Can you work these out from the model? Positions are in its coordinate system, mm. A direction names the side the tool comes from. Give positions to 0.01 mm unless a question says otherwise; leave off trailing zeros. Write each loop counter-clockwise with the first axis right and the second up, starting at its lowest first coordinate (ties: lowest second). Pieces come first, ordered by that corner, then holes. Notation, with made-up numbers: (26, 10) -> (73, 10) arc R10 ccw to (73, 28) -> close; hole circle Ø6 at (-7.5, 48). An arc over 180 degrees is marked (long way). Answer as CSV lines item,"result". Start each with the question number.
1. I need wall thicknesses on line 1 (X direction, y = -6.5, z = 0.5); line 2 (X direction, y = -3.25, z = 101.5); line 3 (Z direction, x = -153, y = -7.5). Which ranges of each line are inside material? Lowest first, please. Write a range as [from, to].
2. If we mould it in two halves opening along Z, with no side actions, what happens to faces 5 (the face through (-297, -6, 162)), 6 (the face through (-451.677, -5.916, -131.161)), 7 (the face through (-230, 0, 110))? For each: pulls with the +Z half, pulls with the -Z half, needs draft (parallel to the pull), parting line crosses it, or undercut.
3. If we section it at B-B on x = -280.5: Write out the boundary of the cut face in (y, z), plus the area to 3 significant figures.
4. If we section it at C-C on y = -3.75: Count the separate pieces of the cut face and the enclosed holes in it, plus the area to 3 significant figures.
5. I'm going to push flat-ended pins straight in: P1, Ø9, axis at x = -303.32, z = 145, coming from the -Y side; P2, Ø3, axis at y = -4.5, z = 82.5, coming from the +X side; P3, Ø5, axis at y = -1, z = -123.5, coming from the +X side; P4, Ø12, axis at x = -200.87, z = 102.3, coming from the -Y side. Where does each tip first touch, or does it pass through?
6. On a 3-axis mill with a long thin cutter (end or side, diameter ignored), from which of +Z, -Z, +X, -X, +Y, -Y can I reach the whole of each face in a straight line? I mean faces 1 (the face through (-453.75, -3.94, 0.55)), 2 (the face through (-269, -8, -119)), 3 (the face through (-151.377, -5.916, 131.009)), 4 (the face through (-452, -5.92, 132.01)). Say none if no direction works.
7. If we section it at D-D on z = -134.5: Write out the boundary of the cut face in (x, y), plus the area to 3 significant figures.
8. If we section it at A-A on z = 145: Write out the boundary of the cut face in (x, y).
```python
from build123d import *

# Parameters (mm, degrees)
F0_R     = 161
F0_R_2   = 5.127079
F0_R_3   = 123
F1_DEPTH = 8
F2_DEPTH = 12


with BuildPart() as f1:
    # F0 (on Front) → F1 (new body)
    with BuildSketch(Plane.XZ):
        with Locations((-303.629764, 0)):
            Circle(F0_R)
        with Locations((-405.93836, -102.751891)):
            Circle(F0_R_2, mode=Mode.SUBTRACT)
        with Locations((-303.317233, -145)):
            Circle(F0_R_2, mode=Mode.SUBTRACT)
        with Locations((-201.317497, -102.748236)):
            Circle(F0_R_2, mode=Mode.SUBTRACT)
        with Locations((-158.629764, -0.304881)):
            Circle(F0_R_2, mode=Mode.SUBTRACT)
        with Locations((-448.629764, 0.323695)):
            Circle(F0_R_2, mode=Mode.SUBTRACT)
        with Locations((-405.930929, 102.75929)):
            Circle(F0_R_2, mode=Mode.SUBTRACT)
        with Locations((-303.629764, 0)):
            Circle(F0_R_3, mode=Mode.SUBTRACT)
        with Locations((-303.317233, 145)):
            Circle(F0_R_2, mode=Mode.SUBTRACT)
        with Locations((-200.870767, 102.301459)):
            Circle(F0_R_2, mode=Mode.SUBTRACT)
    extrude(amount=F1_DEPTH)

    # F0 (on Front) → F2 (join)
    with BuildSketch(Plane.XZ):
        with BuildLine():
            Line((-135.525019, 162), (-463.432019, 162))
            Line((-463.432019, 162), (-440.246351, 101.172665))
            ThreePointArc((-440.246351, 101.172665), (-473.629764, 0), (-440.246351, -101.172665))
            Line((-440.246351, -101.172665), (-463.432019, -162))
            Line((-463.432019, -162), (-135.518019, -162))
            Line((-135.518019, -162), (-166.787395, -100.867071))
            ThreePointArc((-166.787395, -100.867071), (-133.629764, 0.003823), (-166.791931, 100.873225))
            Line((-166.791931, 100.873225), (-135.525019, 162))
        make_face()
        with Locations((-303.629764, 0)):
            Circle(F0_R, mode=Mode.SUBTRACT)
    extrude(amount=F2_DEPTH)


solid = f1.part
```
Computed values:
1,line 1,"x = [-473.63, -453.75], [-443.51, -426.63], [-180.63, -163.69], [-153.57, -133.63]"
1,line 2,"x = [-440.37, -410.9], [-400.96, -373.1], [-234.15, -205.93], [-195.81, -166.47]"
1,line 3,"z = [-162, -127.82], [-78.81, 78.81], [127.84, 162]"
2,face 5,"pulls with the +Z half"
2,face 6,"undercut"
2,face 7,"needs draft"
3,outline,"(-12, -162) -> (0, -162) -> (0, -120.81) -> (-8, -120.81) -> (-8, -159.33) -> (-12, -159.33) -> close; (-12, 159.33) -> (-8, 159.33) -> (-8, 120.81) -> (0, 120.81) -> (0, 162) -> (-12, 162) -> close"
3,area,"680 mm2"
4,separate pieces,"1"
4,enclosed holes,"9"
4,area,"52,900 mm2"
5,P1,"passes through"
5,P2,"stops at x = -154.17"
5,P3,"stops at x = -153.93"
5,P4,"stops at y = -8"
6,face 1,"+Y, -Y"
6,face 2,"-Y"
6,face 3,"+X, +Y, -Y"
6,face 4,"-X, +Y, -Y"
7,outline,"(-452.95, -12) -> (-392.12, -12) -> (-392.12, -8) -> (-215.14, -8) -> (-215.14, -12) -> (-149.58, -12) -> (-149.58, 0) -> (-452.95, 0) -> close"
7,area,"2,930 mm2"
8,outline,"(-456.95, -12) -> (-373.6, -12) -> (-373.6, -8) -> (-308.44, -8) -> (-308.44, 0) -> (-456.95, 0) -> close; (-298.19, -8) -> (-233.66, -8) -> (-233.66, -12) -> (-144.22, -12) -> (-144.22, 0) -> (-298.19, 0) -> close"
